For this review, take the finished solid that the model builds, in its own axes (mm). Round coordinates to 2 decimals unless told otherwise and drop trailing zeros. Write each loop counter-clockwise with the first axis right and the second up, starting at its lowest first coordinate (ties: lowest second). Pieces come first, ordered by that corner, then holes. Notation, with made-up numbers: M 62,87.5 L 90,87.5 A3 cw 90,91.5 Z; hole C 88.5,7 d8. An arc over 180 degrees is marked long. Write each question's results on one line, items separated by ' | '. Start each with the question number.
```python
from build123d import *

# Parameters (mm, degrees)
SKETCH1_W          = 36.5
SKETCH1_H          = 37
EXTRUDE1_DEPTH     = 0.5
CUT_EXTRUDE1_DEPTH = 39.591611783
LPATTERN1_COUNT    = 4
LPATTERN1_PITCH    = 8


with BuildPart() as part:
    # Sketch1 → Extrude1 (new body)
    with BuildSketch(Plane.XY):
        with Locations((0, 15.5)):
            Rectangle(SKETCH1_W, SKETCH1_H)
    extrude(amount=EXTRUDE1_DEPTH)

    # Sketch2 → Cut-Extrude1 (cut, through all)
    with BuildSketch(Plane(origin=(0, 0, 0), x_dir=(-1, 0, 0), z_dir=(0, 0, -1))):
        with BuildLine():
            Line((-15.238638874, 23.185419265), (-9.926046829, 21.761914517))
            ThreePointArc((-9.926046829, 21.761914517), (-7.170370869, 23.352904774), (-8.761361126, 26.108580735))
            Line((-8.761361126, 26.108580735), (-14.073953171, 27.532085483))
            ThreePointArc((-14.073953171, 27.532085483), (-16.829629131, 25.941095226), (-15.238638874, 23.185419265))
        make_face()
        with BuildLine():
            Line((-2.75, 21.75), (2.75, 21.75))
            ThreePointArc((2.75, 21.75), (5, 24), (2.75, 26.25))
            Line((2.75, 26.25), (-2.75, 26.25))
            ThreePointArc((-2.75, 26.25), (-5, 24), (-2.75, 21.75))
        make_face()
        with BuildLine():
            Line((9.926046829, 21.761914517), (15.238638874, 23.185419265))
            ThreePointArc((15.238638874, 23.185419265), (16.829629131, 25.941095226), (14.073953171, 27.532085483))
            Line((14.073953171, 27.532085483), (8.761361126, 26.108580735))
            ThreePointArc((8.761361126, 26.108580735), (7.170370869, 23.352904774), (9.926046829, 21.761914517))
        make_face()
    cut_extrude1 = extrude(amount=-CUT_EXTRUDE1_DEPTH, mode=Mode.SUBTRACT)

    # LPattern1: Cut-Extrude1 ×4
    with Locations(*[(0, -i * LPATTERN1_PITCH, 0) for i in range(1, LPATTERN1_COUNT)]):
        add(cut_extrude1, mode=Mode.SUBTRACT)


solid = part.part
```
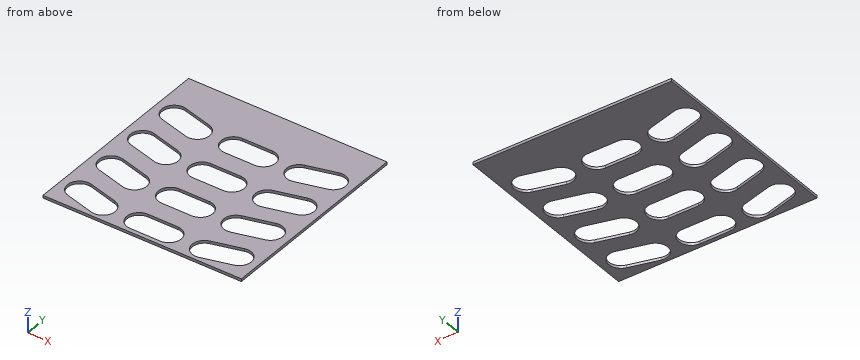
Item 1: We need section A-A on y = 24. State the section outline as (x, z) points, then the cut area to 3 significant figures.
Item 2: Insertion check: P1, Ø5, axis at x = 1.5, y = 25.5, coming from the +Z side. The pin has a flat end and moves straight along its axis. Give the tip position at first contact, or say it passes through.
Item 3: For probe 1 along Y at (x, z) = (-2.5, 0.4); probe 2 along Y at (x, z) = (8.5, 0.15); probe 3 along X at (y, z) = (16.5, 0.1), list the stretches that pass through material, from the lowest coordinate up.
Item 4: We need section B-B on z = 0.15. State how many separate pieces and enclosed holes the cut face has, then the cut area to 3 significant figures.
Numbers:
1) outline: M -18.25,0 L -16.45,0 L -16.45,0.5 L -18.25,0.5 Z; M -7.09,0 L -5,0 L -5,0.5 L -7.09,0.5 Z; M 5,0 L 7.09,0 L 7.09,0.5 L 5,0.5 Z; M 16.45,0 L 18.25,0 L 18.25,0.5 L 16.45,0.5 Z | area: 3.89 mm^2
2) P1: stops at z = 0.5
3) probe 1: y = -3 to -2.25, 2.25 to 5.75, 10.25 to 13.75, 18.25 to 21.75, 26.25 to 34 | probe 2: y = -3 to -2.15, 2.02 to 5.85, 10.02 to 13.85, 18.02 to 21.85, 26.02 to 34 | probe 3: x = -18.25 to -16.74, -7.17 to -4.94, 4.94 to 7.17, 16.74 to 18.25
4) separate pieces: 1 | enclosed holes: 12 | area: 863 mm^2
